Read the model definition and answer for the solid it produces. Units are mm, in the model's axes. Face numbers are marked on the shaded views. A direction names the side the tool comes from. Coordinates: 2 decimals unless noted, no trailing zeros. Write each loop counter-clockwise with the first axis right and the second up, starting at its lowest first coordinate (ties: lowest second). Pieces come first, ordered by that corner, then holes. Notation, with made-up numbers: M 78.25,-9 L 98.25,-9 A18 cw 98.25,0 Z; hole C 31.5,-0.75 d6. An arc over 180 degrees is marked long. Write item = value, one per line.
from build123d import *

# Parameters (mm, degrees)
SKETCH_1_W          = 68
SKETCH_1_H          = 31
SKETCH_1_W_2        = 62
SKETCH_1_H_2        = 25
EXTRUDE_1_DEPTH     = 20
SKETCH_2_W          = 22
SKETCH_2_H          = 1
CUT_EXTRUDE_1_DEPTH = 6
SKETCH_3_R          = 2
CUT_EXTRUDE_2_DEPTH = 3
EXTRUDE_2_DEPTH     = 3
SKETCH_6_R          = 2
CUT_EXTRUDE_3_DEPTH = 49.37354649
SKETCH_8_R          = 3.25
CUT_EXTRUDE_6_DEPTH = 3
SKETCH_9_W          = 68
SKETCH_9_H          = 31
SKETCH_9_W_2        = 62
SKETCH_9_H_2        = 25
EXTRUDE_3_DEPTH     = 60
EXTRUDE_START       = 3
SKETCH_11_W         = 68
SKETCH_11_H         = 80
SKETCH_11_R         = 2
EXTRUDE_5_DEPTH     = 3
SKETCH_12_R         = 6
CUT_EXTRUDE_7_DEPTH = 3


with BuildPart() as part:
    # 草图1 → 凸台-拉伸1 (new body)
    with BuildSketch(Plane(origin=(0, 0, 0), x_dir=(1, 0, 0), z_dir=(0, 1, 0))):
        Rectangle(SKETCH_1_W, SKETCH_1_H)
        Rectangle(SKETCH_1_W_2, SKETCH_1_H_2, mode=Mode.SUBTRACT)
    extrude(amount=EXTRUDE_1_DEPTH)

    # 草图2 → 切除-拉伸1 (cut)
    with BuildSketch(Plane(origin=(0, 20, 0), x_dir=(1, 0, 0), z_dir=(0, 1, 0))):
        with Locations((0, 15)):
            Rectangle(SKETCH_2_W, SKETCH_2_H)
    extrude(amount=-CUT_EXTRUDE_1_DEPTH, mode=Mode.SUBTRACT)

    # 草图3 → 切除-拉伸2 (cut)
    with BuildSketch(Plane(origin=(0, 0, -15.5), x_dir=(-1, 0, 0), z_dir=(0, 0, -1))):
        with Locations((-8, 10)):
            Circle(SKETCH_3_R)
        with Locations((8, 10)):
            Circle(SKETCH_3_R)
    extrude(amount=-CUT_EXTRUDE_2_DEPTH, mode=Mode.SUBTRACT)

    # 草图4 → 凸台-拉伸2 (add)
    with BuildSketch(Plane(origin=(0, 0, -15.5), x_dir=(-1, 0, 0), z_dir=(0, 0, -1))):
        Polygon((-11, 14), (-13, 14), (-13, 4), (-11, 4), (11, 4), (13, 4), (13, 14), (11, 14), align=None)
    extrude(amount=EXTRUDE_2_DEPTH)

    # 草图6 → 切除-拉伸3 (cut, symmetric)
    with BuildSketch(Plane.XY.offset(-12.5)):
        with Locations((-8, 10)):
            Circle(SKETCH_6_R)
        with Locations((8, 10)):
            Circle(SKETCH_6_R)
    cut_extrude_3 = extrude(amount=CUT_EXTRUDE_3_DEPTH, both=True, mode=Mode.SUBTRACT)

    # 草图8 → 切除-拉伸6 (cut)
    with BuildSketch(Plane.XY.offset(-12.5)):
        with Locations((-8, 10)):
            Circle(SKETCH_8_R)
        with Locations((8, 10)):
            Circle(SKETCH_8_R)
    extrude(amount=-CUT_EXTRUDE_6_DEPTH, mode=Mode.SUBTRACT)

    # 草图9 → 凸台-拉伸3 (add)
    with BuildSketch(Plane.XZ):
        Rectangle(SKETCH_9_W, SKETCH_9_H)
        Rectangle(SKETCH_9_W_2, SKETCH_9_H_2, mode=Mode.SUBTRACT)
    extrude(amount=EXTRUDE_3_DEPTH)

    # 草图11 → 凸台-拉伸5 (add)
    with BuildSketch(Plane.XY.offset(15.5).offset(EXTRUDE_START)):
        with Locations((0, -20)):
            Rectangle(SKETCH_11_W, SKETCH_11_H)
        with Locations((-8, 10)):
            Circle(SKETCH_11_R, mode=Mode.SUBTRACT)
        with Locations((8, 10)):
            Circle(SKETCH_11_R, mode=Mode.SUBTRACT)
    extrude(amount=-EXTRUDE_5_DEPTH)

    # 草图12 → 切除-拉伸7 (cut)
    with BuildSketch(Plane(origin=(0, 0, 12.5), x_dir=(-1, 0, 0), z_dir=(0, 0, -1))):
        with Locations((-8, 10)):
            Circle(SKETCH_12_R)
        with Locations((8, 10)):
            Circle(SKETCH_12_R)
    cut_extrude_7 = extrude(amount=-CUT_EXTRUDE_7_DEPTH, mode=Mode.SUBTRACT)

    # 镜向1: 切除-拉伸3, 切除-拉伸7 across plane
    add(cut_extrude_3.mirror(Plane.ZX.offset(-20)), mode=Mode.SUBTRACT)
    add(cut_extrude_7.mirror(Plane.ZX.offset(-20)), mode=Mode.SUBTRACT)


solid = part.part
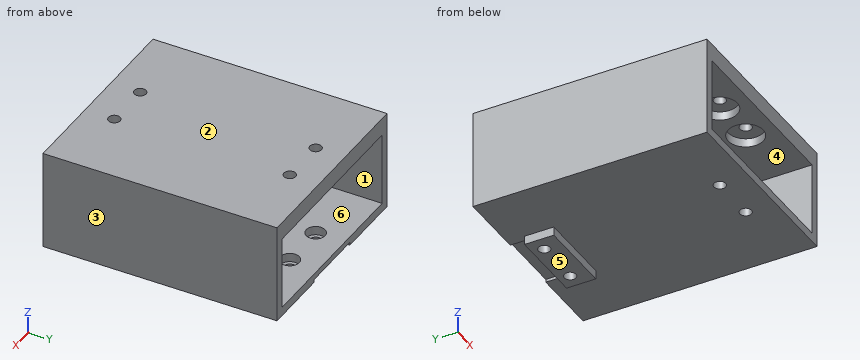
Item 1: Find section B-B (z = -2.5). Determine the outline of the cut face in (x, y).
Worked answers:
outline = M -34,-60 L -31,-60 L -31,20 L -34,20 Z; M 31,-60 L 34,-60 L 34,20 L 31,20 Z
Item 2: Consider line 1 along Y through (x, z) = (8, -13); line 2 along Y through (x, z) = (-8, 17); line 3 along X through (y, z) = (-50, 13). Determine where each line is inside the solid, lowest interval first. Write a range as from..to.
Worked answers:
line_1 = -60..-52, -48..6.75, 13.25..20
line_2 = -60..-52, -48..8, 12..20
line_3 = -34..-14, -2..2, 14..34
Item 3: Find section A-A (y = -50). State how many separate pieces and enclosed holes the cut face has, and give its area (3 significant figures).
Worked answers:
separate_pieces = 4
enclosed_holes = 0
area = 642 mm²
Item 4: Flat-ended cylindrical pins translate along their axes: pin 1 (6.5 mm diameter, centred on x = -8, y = -50, fed in from +Z); pin 2 (12 mm diameter, centred on x = 13, z = 5.5, fed in from +Y); pin 3 (5 mm diameter, centred on x = 1.5, y = -32.5, fed in from -Z). Find the tip coordinate at first contact, or state that the pin passes through.
Worked answers:
pin_1 = 18.5
pin_2 = through
pin_3 = -15.5
Item 5: For a pull along Z with two mould halves and no side action, classify the marked faces 1, 2, 3 and 4 as released by +Z, released by -Z, zero draft, split by the parting line, or undercut.
Worked answers:
face_1 = undercut
face_2 = released by +Z
face_3 = zero draft
face_4 = undercut
Item 6: Find section D-D (y = -6.5). Determine the outline of the cut face in (x, z), and give its area (3 significant figures).
Worked answers:
outline = M -34,-15.5 L 34,-15.5 L 34,18.5 L -34,18.5 Z; hole M -31,-12.5 L 31,-12.5 L 31,12.5 L -31,12.5 Z
area = 762 mm²
Item 7: Which of the six approach directions +Z, -Z, +X, -X, +Y, -Y give full straight-line access (tool end or side, diameter ignored) to the marked faces 5 and 6?
Worked answers:
face_5 = -Z, +X, -X, +Y, -Y
face_6 = +Y, -Y
